Part model, mm, in its own coordinate system. A direction names the side the tool comes from. Give positions to 0.01 mm unless a question says otherwise; leave off trailing zeros. Order: outer loops, then holes, each group sorted by start corner. A loop starts at its lowest first (then second) coordinate and runs counter-clockwise, first axis right, second up. Notation, with made-up numbers: M 25,-34 L 36,-34 A10 ccw 36,-23 Z; hole C 16,-13 d1. An arc over 180 degrees is marked long. One line per question, with ' | ' between items.
```python
from build123d import *

# Parameters (mm, degrees)
SKETCH1_W           = 36
SKETCH1_H           = 34
BOSS_EXTRUDE6_DEPTH = 1
SKETCH7_R           = 12
CUT_EXTRUDE1_DEPTH  = 1
EXTRUDE_THIN1_DEPTH = 15
SKETCH10_W          = 6.466905847
SKETCH10_H          = 48.062044255
CUT_EXTRUDE2_DEPTH  = 29.948229652
SKETCH11_W          = 36
SKETCH11_H          = 1
EXTRUDE_THIN2_DEPTH = 14
FILLET3_R           = 1.5
SKETCH12_R          = 1.5
BOSS_EXTRUDE7_DEPTH = 5
SKETCH13_R          = 1
CUT_EXTRUDE3_DEPTH  = 5


with BuildPart() as part:
    # Sketch1 → Boss-Extrude6 (new body)
    with BuildSketch(Plane.YZ):
        Rectangle(SKETCH1_W, SKETCH1_H)
    extrude(amount=BOSS_EXTRUDE6_DEPTH)

    # Sketch7 → Cut-Extrude1 (cut)
    with BuildSketch(Plane.YZ.offset(1)):
        with Locations(Location((0, 3, 0), (0, 0, 270))):
            Circle(SKETCH7_R)
    extrude(amount=-CUT_EXTRUDE1_DEPTH, mode=Mode.SUBTRACT)

    # Sketch9 → Extrude-Thin1 (add)
    with BuildSketch(Plane(origin=(1, 0, 0), x_dir=(0, 0, -1), z_dir=(1, 0, 0))):
        Polygon((17, -18), (-17, -18), (-17, 18), (17, 18), (17, 17), (-16, 17), (-16, -17), (17, -17), align=None)
    extrude(amount=-EXTRUDE_THIN1_DEPTH)

    # Sketch10 → Cut-Extrude2 (cut, through all)
    with BuildSketch(Plane(origin=(1, 0, 0), x_dir=(0, 0, -1), z_dir=(1, 0, 0))):
        with Locations((14.233452923, -0.025867623)):
            Rectangle(SKETCH10_W, SKETCH10_H)
    extrude(amount=-CUT_EXTRUDE2_DEPTH, mode=Mode.SUBTRACT)

    # Sketch11 → Extrude-Thin2 (add)
    with BuildSketch(Plane.YZ):
        with Locations((0, -10.5)):
            Rectangle(SKETCH11_W, SKETCH11_H)
    extrude(amount=-EXTRUDE_THIN2_DEPTH)

    # Fillet3
    fillet3_edges = [part.edges().sort_by_distance(p)[0] for p in [
        (-6.5, 18, -11),
        (-6.5, -18, -11),
        (-6.5, -18, 17),
        (-6.5, 18, 17),
    ]]
    fillet(fillet3_edges, radius=FILLET3_R)

    # Sketch12 → Boss-Extrude7 (add)
    with BuildSketch(Plane.YZ):
        with Locations(Location((-14.5, 3.5, 0), (0, 0, 270))):
            Circle(SKETCH12_R)
    boss_extrude7 = extrude(amount=-BOSS_EXTRUDE7_DEPTH)

    # Sketch13 → Cut-Extrude3 (cut)
    with BuildSketch(Plane(origin=(-5, 0, 0), x_dir=(0, -1, 0), z_dir=(-1, 0, 0))):
        with Locations(Location((14.5, 3.5, 0), (0, 0, 90))):
            Circle(SKETCH13_R)
    cut_extrude3 = extrude(amount=-CUT_EXTRUDE3_DEPTH, mode=Mode.SUBTRACT)

    # Mirror1: Boss-Extrude7, Cut-Extrude3 across plane
    add(boss_extrude7.mirror(Plane.ZX))
    add(cut_extrude3.mirror(Plane.ZX), mode=Mode.SUBTRACT)


solid = part.part
```
1. Tool access for faces 4 (the cylindrical face through (-2.535, -15.476, 3.283)), 5 (the flat face through (-6, 18, 3)): list every direction of +Z, -Z, +X, -X, +Y, -Y with a clear straight run to the whole face (end or side of a thin tool).
Worked out:
face 4: -X | face 5: +Z, -Z, +X, -X, +Y
2. Probe L1, parallel to Y at x = -3.35, z = 3.5; L2, parallel to Z at x = -12.75, y = -16; L3, parallel to Y at x = -3, z = -3.5. List the from-to ranges inside material, lowest first. Write a range as from..to.
Worked out:
L1: y = -18..-17, -16..-15.5, -13.5..-13, 13..13.5, 15.5..16, 17..18 | L2: z = -11..-10, 16..17 | L3: y = -18..-17, 17..18
3. Slice it at C-C on x = -12.5. Give the cut face in (y, z).
Worked out:
outline: M -18,-9.5 A1.5 ccw -16.5,-11 L 16.5,-11 A1.5 ccw 18,-9.5 L 18,15.5 A1.5 ccw 16.5,17 L -16.5,17 A1.5 ccw -18,15.5 Z; hole M -17,-10 L 17,-10 L 17,16 L -17,16 Z
4. Slice it at B-B on z = -7.75. Give the cut face in (x, y), then the cut area to 3 significant figures.
Worked out:
outline: M -14,-18 L 1,-18 L 1,-5.33 L 0,-5.33 L 0,-17 L -14,-17 Z; M -14,17 L 0,17 L 0,5.33 L 1,5.33 L 1,18 L -14,18 Z | area: 53.3 mm2
5. Mould opens along Z. For faces 1 (the cylindrical face through (-6.6, -17.57, 16.55)), 2 (the cylindrical face through (-2.535, 15.476, 3.283)), 3 (the flat face through (-14, 0.1, -10.5)) say: released by +Z, released by -Z, zero draft, split by the parting line, or undercut.
Worked out:
face 1: released by +Z | face 2: undercut | face 3: zero draft
6. Slice it at D-D on y = 14.5. Give the cut face in (x, z), then the cut area to 3 significant figures.
Worked out:
outline: M -14,-11 L 1,-11 L 1,17 L -14,17 L -14,16 L 0,16 L 0,5 L -5,5 L -5,4.5 L 0,4.5 L 0,2.5 L -5,2.5 L -5,2 L 0,2 L 0,-10 L -14,-10 Z | area: 61.0 mm2
7. Slice it at A-A on y = 0. Give the cut face in (x, z), then the cut area to 3 significant figures.
Worked out:
outline: M -14,-11 L 1,-11 L 1,-9 L 0,-9 L 0,-10 L -14,-10 Z; M -14,16 L 0,16 L 0,15 L 1,15 L 1,17 L -14,17 Z | area: 32.0 mm2
8. Drop flat-ended pins along their axis: pin 1 (2.5 mm diameter, centred on y = 15, z = 3.5, fed in from -X); pin 2 (6 mm diameter, centred on y = -1.5, z = -6, fed in from -X). Give the stop position or say it passes through.
Worked out:
pin 1: stops at x = -5 | pin 2: stops at x = 0
